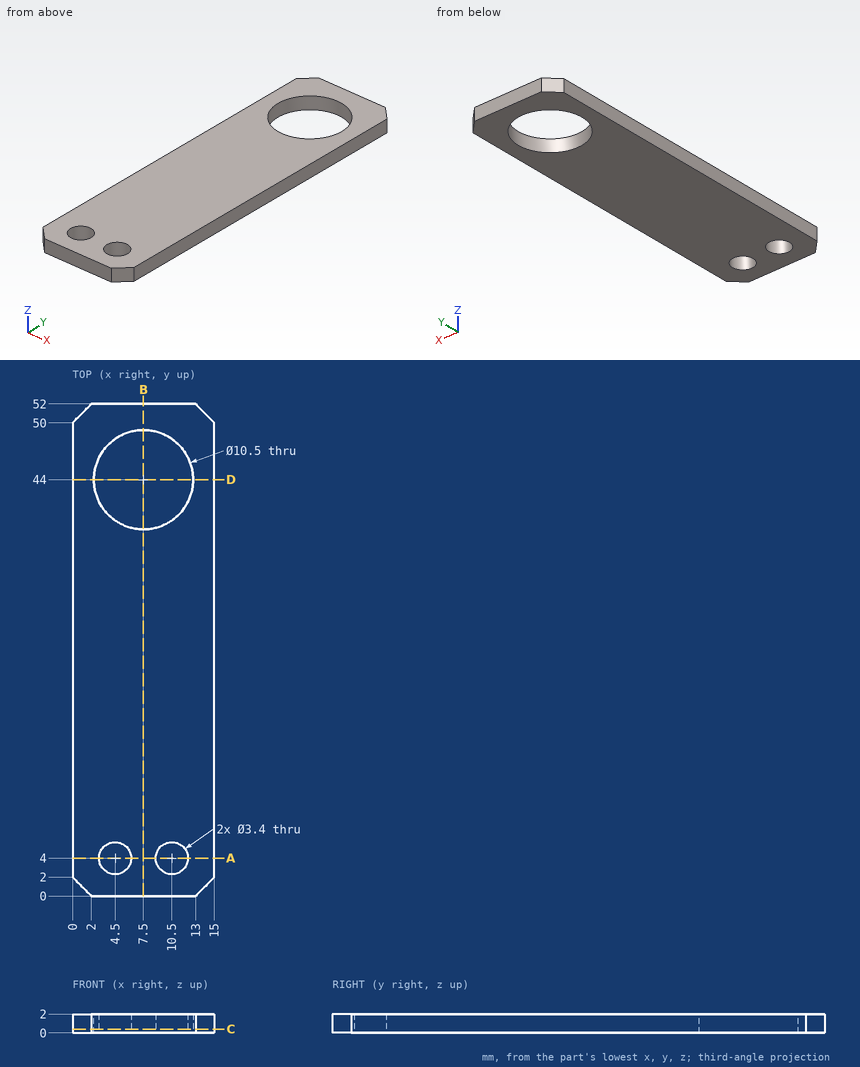
For this review, use the dimensioned drawing (mm, ordinates from the lowest corner) and the shaded views. Round coordinates to 2 decimals unless told otherwise and drop trailing zeros. Write each loop counter-clockwise with the first axis right and the second up, starting at its lowest first coordinate (ties: lowest second). Pieces come first, ordered by that corner, then holes. Notation, with made-up numbers: (25.5, 78.5) - (72.5, 78.5) arc R23 ccw to (72.5, 87.5) - close; hole circle Ø7 at (33, 21). An arc over 180 degrees is marked (long way). One line per item, written item: value. Start each with the question number.
1. Consider section D-D on y = 44. Write out the cut boundary in (x, z), and give its area (3 significant figures).
2. To check wall thickness, follow L1, parallel to X at y = 4, z = 1.3; L2, parallel to Y at x = 7.5, z = 0.65; L3, parallel to X at y = 44, z = 0.7. State the ranges of each line that lie inside material, in increasing order. Write a range as from..to.
3. Clearance check with flat-ended pins moving along their axes: P1, Ø6, axis at x = 12, y = 23.5, coming from the -Z side; P2, Ø2, axis at x = 10.5, y = 4, coming from the -Z side. State where each tip first meets the part, or that it passes through.
4. Consider section A-A on y = 4. Write out the cut boundary in (x, z).
5. Consider section B-B on x = 7.5. Write out the cut boundary in (y, z), and give its area (3 significant figures).
6. Consider section C-C on z = 0.4. Write out the cut boundary in (x, y), and give its area (3 significant figures).
Checks:
1. outline: (0, 0) - (2.25, 0) - (2.25, 2) - (0, 2) - close; (12.75, 0) - (15, 0) - (15, 2) - (12.75, 2) - close
1. area: 9.00 mm^2
2. L1: x = 0..2.8, 6.2..8.8, 12.2..15
2. L2: y = 0..38.75, 49.25..52
2. L3: x = 0..2.25, 12.75..15
3. P1: stops at z = 0
3. P2: passes through
4. outline: (0, 0) - (2.8, 0) - (2.8, 2) - (0, 2) - close; (6.2, 0) - (8.8, 0) - (8.8, 2) - (6.2, 2) - close; (12.2, 0) - (15, 0) - (15, 2) - (12.2, 2) - close
5. outline: (0, 0) - (38.75, 0) - (38.75, 2) - (0, 2) - close; (49.25, 0) - (52, 0) - (52, 2) - (49.25, 2) - close
5. area: 83.0 mm^2
6. outline: (0, 2) - (2, 0) - (13, 0) - (15, 2) - (15, 50) - (13, 52) - (2, 52) - (0, 50) - close; hole circle Ø10.5 at (7.5, 44); hole circle Ø3.4 at (4.5, 4); hole circle Ø3.4 at (10.5, 4)
6. area: 667 mm^2
